The listing builds one solid part. Answer for the finished solid, in the listing's coordinates (mm). Face numbers are marked on the shaded views. Give positions to 0.01 mm unless a question says otherwise; leave off trailing zeros. Write each loop counter-clockwise with the first axis right and the second up, starting at its lowest first coordinate (ties: lowest second). Pieces come first, ordered by that corner, then holes. Notation, with made-up numbers: (23, 89.25) - (41, 89.25) arc R18 ccw to (41, 93.25) - close; hole circle Ø2 at (25, 6.25). An arc over 180 degrees is marked (long way). Answer as CSV lines item,"result". Start each with the question number.
(1) Find section A-A (y = -1). State how many separate pieces and enclosed holes the cut face has, then the cut area to 3 significant figures.
(2) Each of these flat-tipped pins is pushed along its axis until it touches: pin 1 Ø0.5 at (y, z) = (-2, 0) entering from +X; pin 2 Ø1.5 at (x, y) = (-0.5, -2.5) entering from -Z; pin 3 Ø0.5 at (x, y) = (0, -2.5) entering from +Z. Where does it stop, or does it pass through?
(3) Find section C-C (x = 1.1). Write down the section's boundary in (y, z), then the cut area to 3 significant figures.
(4) For a pull along Z with two mould halves and no side action, classify the marked faces 1, 2 and 3 as pulls with the +Z half, pulls with the -Z half, needs draft (parallel to the pull), parting line crosses it, or undercut.
(5) Straight lines are drawn through the part: probe 1 along Y at (x, z) = (0.15, -1); probe 2 along Y at (x, z) = (0.8, 0.5). For each, find the intervals that lie inside material, in ascending order.
(6) Find section D-D (z = 5.25). Write down the section's boundary in (x, y), then the cut area to 3 significant figures.
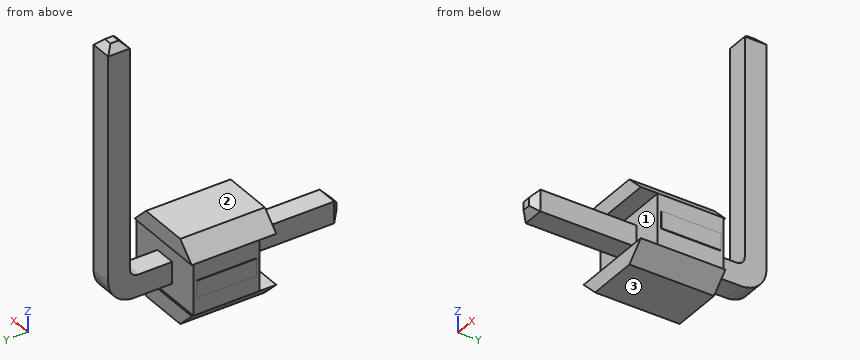
from build123d import *
from OCP.BRepFilletAPI import BRepFilletAPI_MakeFillet

# Parameters (mm, degrees)
BOSS_EXTRUDE1_DEPTH = 0.32
FILLET1_R1          = 0.75
FILLET1_R2          = 0.25
BOSS_EXTRUDE3_DEPTH = 1.25
CHAMFER1_SIZE       = 0.5
SKETCH3_W           = 0.5
SKETCH3_H           = 1.75
BOSS_EXTRUDE4_DEPTH = 1.27
CHAMFER2_SIZE       = 0.2


with BuildPart() as part:
    # Sketch1 → Boss-Extrude1 (new, symmetric)
    with BuildSketch(Plane(origin=(0, 0, 0), x_dir=(0, 0, -1), z_dir=(1, 0, 0))):
        Polygon((-7.25, 2.45), (-0.32, 2.45), (-0.32, -3.79), (0.32, -3.79), (0.32, 3.09), (-7.25, 3.09), align=None)
    extrude(amount=BOSS_EXTRUDE1_DEPTH, both=True)

    # Fillet1: one fillet with a radius per group of edges: ONE call of the kernel's fillet builder (fillet() takes one radius for all edges)
    fillet1_edges_1 = [part.edges().sort_by_distance(p)[0] for p in [
        (0, 3.09, -0.32),
    ]]
    fillet1_edges_2 = [part.edges().sort_by_distance(p)[0] for p in [
        (0, 2.45, 0.32),
    ]]
    fillet1 = BRepFilletAPI_MakeFillet(part.part.solid().wrapped)
    for e in fillet1_edges_1:
        fillet1.Add(FILLET1_R1, e.wrapped)
    for e in fillet1_edges_2:
        fillet1.Add(FILLET1_R2, e.wrapped)
    add(Compound.cast(fillet1.Shape()), mode=Mode.REPLACE)

    # Sketch2 → Boss-Extrude3 (add, symmetric)
    with BuildSketch(Plane(origin=(0, 0, 0), x_dir=(0, -1, 0), z_dir=(1, 0, 0))):
        Polygon((-1.25, 1.25), (1.25, 1.25), (1.25, 0.75), (0.75, 0.75), (0.75, -0.75), (1.25, -0.75), (1.25, -1.25), (-1.25, -1.25), (-1.25, -0.75), (-1.2, -0.75), (-1.2, 0.75), (-1.25, 0.75), align=None)
    extrude(amount=BOSS_EXTRUDE3_DEPTH, both=True)

    # Chamfer1
    chamfer1_edges = [part.edges().sort_by_distance(p)[0] for p in [
        (1.25, 0, 1.25),
        (1.25, 0, -1.25),
        (-1.25, 0, 1.25),
        (-1.25, 0, -1.25),
    ]]
    chamfer(chamfer1_edges, length=CHAMFER1_SIZE - 0.0001)  # a hair under: the kernel refuses the full size

    # Sketch3 → Boss-Extrude4 (add, symmetric)
    with BuildSketch(Plane(origin=(0, 0, 0), x_dir=(0, 0, -1), z_dir=(1, 0, 0))):
        with Locations((0, 0.225)):
            Rectangle(SKETCH3_W, SKETCH3_H)
    extrude(amount=BOSS_EXTRUDE4_DEPTH, both=True)

    # Chamfer2
    chamfer2_edges = [part.edges().sort_by_distance(p)[0] for p in [
        (0, 3.09, 7.25),
        (0, -3.79, -0.32),
        (0, -3.79, 0.32),
        (0, 2.45, 7.25),
        (0.32, -3.79, 0),
        (0.32, 2.77, 7.25),
        (-0.32, -3.79, 0),
        (-0.32, 2.77, 7.25),
    ]]
    chamfer(chamfer2_edges, length=CHAMFER2_SIZE)


solid = part.part
Result set:
1,separate pieces,"3"
1,enclosed holes,"0"
1,area,"2.41 mm^2"
2,pin 1,"x = 0.32"
2,pin 2,"z = -0.32"
2,pin 3,"z = 0.32"
3,outline,"(-1.25, -0.9) - (1.25, -0.9) - (1.25, -0.75) - (1.2, -0.75) - (1.2, 0.75) - (1.25, 0.75) - (1.25, 0.9) - (-1.25, 0.9) - (-1.25, 0.75) - (-0.75, 0.75) - (-0.75, -0.75) - (-1.25, -0.75) - close"
3,area,"3.68 mm^2"
4,face 1,"undercut"
4,face 2,"pulls with the +Z half"
4,face 3,"pulls with the -Z half"
5,probe 1,"-1.25 to 1.25"
5,probe 2,"-0.75 to 1.2"
6,outline,"(-0.32, 2.45) - (0.32, 2.45) - (0.32, 3.09) - (-0.32, 3.09) - close"
6,area,"0.410 mm^2"
